```python
from build123d import *

# Parameters (mm, degrees)
SKETCH_1_R      = 1.5
EXTRUDE_1_DEPTH = 2


with BuildPart() as part:
    # 草图1 → 凸台-拉伸1 (new body)
    with BuildSketch(Plane.XY):
        Polygon((16.993865071, 15.9), (16.993865071, 20), (-16.993865071, 20), (-16.993865071, 15.9), (-16.993865071, -14), (-18.993865071, -14), (-18.993865071, -19), (-16.993865071, -19), (-16.993865071, -22.5), (-14.493865071, -22.5), (-14.493865071, -21), (-11.893865071, -21), (-11.893865071, -22.5), (-8.893865071, -22.5), (-8.893865071, -25.5), (-11.893865071, -25.5), (-11.893865071, -27), (-14.493865071, -27), (-14.493865071, -25.5), (-16.993865071, -25.5), (-16.993865071, -29), (-18.993865071, -29), (-18.993865071, -34), (-16.993865071, -34), (-16.993865071, -84), (-18.993865071, -84), (-18.993865071, -89), (-16.993865071, -89), (-16.993865071, -92.5), (-14.493865071, -92.5), (-14.493865071, -91), (-11.893865071, -91), (-11.893865071, -92.5), (-8.893865071, -92.5), (-8.893865071, -95.5), (-11.893865071, -95.5), (-11.893865071, -97), (-14.493865071, -97), (-14.493865071, -95.5), (-16.993865071, -95.5), (-16.993865071, -99), (-18.993865071, -99), (-18.993865071, -104), (-16.993865071, -104), (-16.993865071, -108), (-0.721190694, -108), (0, -109.5), (0.721190694, -108), (16.993865071, -108), (69.553865071, -108), (69.553865071, -105), (69.553865071, -99), (18.993865071, -84), (16.993865071, -84), (16.993865071, -34), (18.993865071, -34), (18.993865071, -29), (16.993865071, -29), (16.993865071, -25.5), (14.493865071, -25.5), (14.493865071, -27), (11.893865071, -27), (11.893865071, -25.5), (8.893865071, -25.5), (8.893865071, -22.5), (11.893865071, -22.5), (11.893865071, -21), (14.493865071, -21), (14.493865071, -22.5), (16.993865071, -22.5), (16.993865071, -19), (18.993865071, -19), (71.993865071, 0.9), (71.993865071, 15.9), align=None)
        with Locations((0, -104)):
            Circle(SKETCH_1_R, mode=Mode.SUBTRACT)
        Circle(SKETCH_1_R, mode=Mode.SUBTRACT)
        with Locations((0, 10)):
            Circle(SKETCH_1_R, mode=Mode.SUBTRACT)
        with Locations((50, -104)):
            Circle(SKETCH_1_R, mode=Mode.SUBTRACT)
        with BuildLine():
            Line((13.9, -105.15), (8.6, -105.15))
            ThreePointArc((8.6, -105.15), (8.123654403, -104), (8.6, -102.85))
            Line((8.6, -102.85), (13.9, -102.85))
            Line((13.9, -102.85), (13.9, -105.15))
        make_face(mode=Mode.SUBTRACT)
        with BuildLine():
            Line((-13.9, -102.85), (-8.6, -102.85))
            ThreePointArc((-8.6, -102.85), (-8.123654403, -104), (-8.6, -105.15))
            Line((-8.6, -105.15), (-13.9, -105.15))
            Line((-13.9, -105.15), (-13.9, -102.85))
        make_face(mode=Mode.SUBTRACT)
        with BuildLine():
            Line((63.9, -105.15), (58.6, -105.15))
            ThreePointArc((58.6, -105.15), (58.123654403, -104), (58.6, -102.85))
            Line((58.6, -102.85), (63.9, -102.85))
            Line((63.9, -102.85), (63.9, -105.15))
        make_face(mode=Mode.SUBTRACT)
    extrude(amount=EXTRUDE_1_DEPTH)


solid = part.part
```
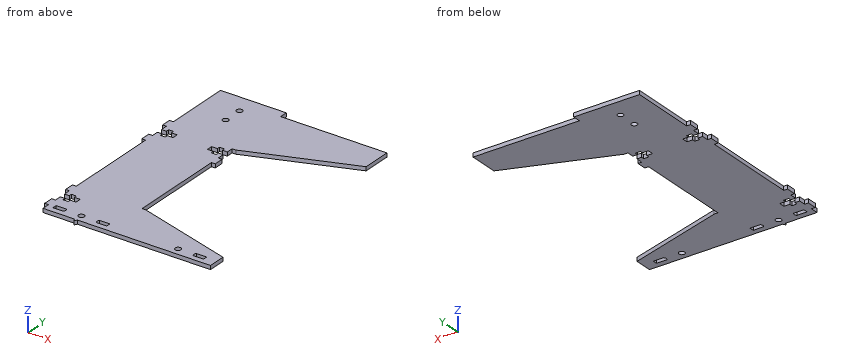
Here's how the part is built. I have some questions about the finished solid (model axes, mm). Coordinates: 2 decimals unless noted, no trailing zeros. Order: outer loops, then holes, each group sorted by start corner. A loop starts at its lowest first (then second) coordinate and runs counter-clockwise, first axis right, second up. Notation, with made-up numbers: (17, 11.5) - (75, 11.5) arc R14 ccw to (75, 17.5) - close; hole circle Ø9 at (-30.75, 82). An arc over 180 degrees is marked (long way). One line per question, with ' | ' between items. Start each with the question number.
1. If we section it at A-A (y = 10): Write out the boundary of the cut face in (x, z).
2. If we section it at B-B (x = 32): Write out the boundary of the cut face in (y, z), and give its area (3 significant figures).
3. Please list where these lines run through material, in increasing order: line 1 along Y through (x, z) = (-11.5, 0.2); line 2 along X through (y, z) = (-22, 0.75); line 3 along Y through (x, z) = (62, 1.25). Write a range as [from, to].
4. I'm going to push flat-ended pins straight in: pin 1 Ø1 at (y, z) = (3.5, 1) entering from -X; pin 2 Ø0.6 at (x, z) = (11, 0.5) entering from -Y; pin 3 Ø0.6 at (x, z) = (61.5, 1.5) entering from +Y; pin 4 Ø1.5 at (x, y) = (55, -6) entering from -Z. Where does each tip first touch, or does it pass through?
5. If we section it at C-C (z = 1.6): Give the number of separate pieces and of enclosed holes in the cut face, and give its area (3 significant figures).
6. If we section it at D-D (x = 50): Write out the boundary of the cut face in (y, z).
Model answer:
1) outline: (-16.99, 0) - (-1.5, 0) - (-1.5, 2) - (-16.99, 2) - close; (1.5, 0) - (71.99, 0) - (71.99, 2) - (1.5, 2) - close
2) outline: (-108, 0) - (-87.86, 0) - (-87.86, 2) - (-108, 2) - close; (-14.12, 0) - (15.9, 0) - (15.9, 2) - (-14.12, 2) - close | area: 100 mm²
3) line 1: y = [-108, -105.15], [-102.85, -95.5], [-92.5, -25.5], [-22.5, 20] | line 2: x = [-16.99, -14.49], [-11.89, 11.89], [14.49, 16.99] | line 3: y = [-108, -105.15], [-102.85, -96.76], [-2.85, 15.9]
4) pin 1: stops at x = -16.99 | pin 2: stops at y = -108 | pin 3: stops at y = 15.9 | pin 4: stops at z = 0
5) separate pieces: 1 | enclosed holes: 7 | area: 6,510 mm²
6) outline: (-108, 0) - (-105.5, 0) - (-105.5, 2) - (-108, 2) - close; (-102.5, 0) - (-93.2, 0) - (-93.2, 2) - (-102.5, 2) - close; (-7.36, 0) - (15.9, 0) - (15.9, 2) - (-7.36, 2) - close
